For this review, take the finished solid that the model builds, in its own axes (mm). Face numbers are marked on the shaded views. A direction names the side the tool comes from. Round coordinates to 2 decimals unless told otherwise and drop trailing zeros. Write each loop counter-clockwise with the first axis right and the second up, starting at its lowest first coordinate (ties: lowest second). Pieces come first, ordered by that corner, then holes. Notation, with made-up numbers: (79, 67) -> (122, 67) arc R11 ccw to (122, 75) -> close; hole circle Ø3 at (6.5, 85). An arc over 180 degrees is marked (long way). Answer as CSV lines item,"result". Start each with the question number.
Item 1: Take a section at A-A on y = 0. Give the boundary of the cut face in (x, z), then the cut area to 3 significant figures.
Item 2: Wall thickness on probe 1 along Y at (x, z) = (0.5, 2.25); probe 2 along X at (y, z) = (15, 5.25): over which ranges is each line inside the solid? List them lowest first. Write a range as from..to.
Item 3: Machinability: for the marked faces 5 and 6, which of the approach directions +Z, -Z, +X, -X, +Y, -Y give a long, thin tool a straight path to every point of the face, cutting with its end or side? Answer none if there is none.
Item 4: Mouldability with a two-part tool opening along X and no side actions: class the marked faces 1, 2, 3 and 4 as +X half, -X half, draft (parallel to the pull), parting line (faces both ways), or undercut.
Item 5: For pin 1 Ø18.5 at (x, y) = (-3.5, -2) entering from -Z; pin 2 Ø5 at (x, y) = (16, 16) entering from -Z, all flat-tipped, find the tip position at first contact; note any pin that passes through.
Item 6: Take a section at C-C on z = 3. Count the separate pieces of the cut face and the enclosed holes in it, then the cut area to 3 significant figures.
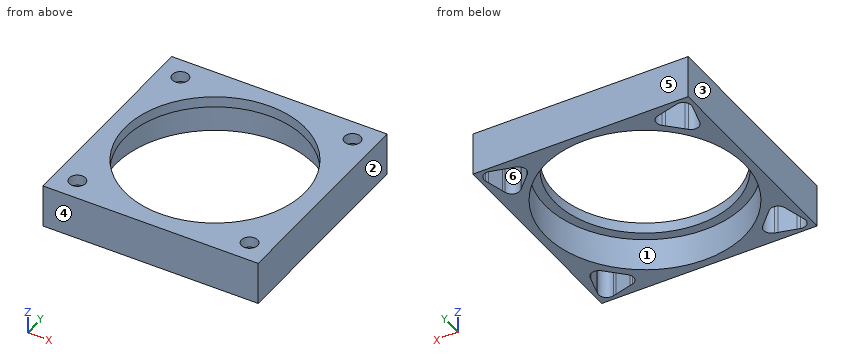
```python
from build123d import *

# Parameters (mm, degrees)
SKETCH_W        = 40
SKETCH_H        = 40
PAD_DEPTH       = 6
POCKET_DEPTH    = 6.001
SKETCH006_R     = 18.5
POCKET001_DEPTH = 6.001
SKETCH007_W     = 40
SKETCH007_H     = 40
SKETCH007_R     = 16.75
SKETCH007_R_2   = 1.5
PAD001_DEPTH    = 2


with BuildPart() as part:
    # Sketch → Pad (new body)
    with BuildSketch(Plane.XY):
        Rectangle(SKETCH_W, SKETCH_H)
    extrude(amount=PAD_DEPTH)

    # Sketch004 (on Face6 of Pad) → Pocket (cut, through all)
    with BuildSketch(Plane.XY.offset(6)):
        with BuildLine():
            Line((12.932774, 15.178139), (15.178139, 12.932774))
            Line((15.178139, 12.932774), (15.586387, 12.524525))
            ThreePointArc((15.586387, 12.524525), (17.035276, 12.136297), (18.095936, 13.196957))
            Line((18.245366, 13.754634), (18.095936, 13.196957))
            Line((18.245366, 13.754634), (19.067226, 16.821861))
            Line((19.067226, 16.821861), (19.216656, 17.379538))
            ThreePointArc((19.216656, 17.379538), (18.828427, 18.828427), (17.379538, 19.216656))
            Line((16.821861, 19.067226), (17.379538, 19.216656))
            Line((16.821861, 19.067226), (13.754634, 18.245366))
            Line((13.754634, 18.245366), (13.196957, 18.095936))
            ThreePointArc((13.196957, 18.095936), (12.136297, 17.035276), (12.524525, 15.586387))
            Line((12.932774, 15.178139), (12.524525, 15.586387))
        make_face()
        with BuildLine():
            Line((13.754634, -18.245366), (16.821861, -19.067226))
            Line((16.821861, -19.067226), (17.379538, -19.216656))
            ThreePointArc((17.379538, -19.216656), (18.828427, -18.828427), (19.216656, -17.379538))
            Line((19.067226, -16.821861), (19.216656, -17.379538))
            Line((19.067226, -16.821861), (18.245366, -13.754634))
            Line((18.245366, -13.754634), (18.095936, -13.196957))
            ThreePointArc((18.095936, -13.196957), (17.035276, -12.136297), (15.586387, -12.524525))
            Line((15.178139, -12.932774), (15.586387, -12.524525))
            Line((15.178139, -12.932774), (12.932774, -15.178139))
            Line((12.932774, -15.178139), (12.524525, -15.586387))
            ThreePointArc((12.524525, -15.586387), (12.136297, -17.035276), (13.196957, -18.095936))
            Line((13.754634, -18.245366), (13.196957, -18.095936))
        make_face()
        with BuildLine():
            Line((-13.754634, 18.245366), (-16.821861, 19.067226))
            Line((-16.821861, 19.067226), (-17.379538, 19.216656))
            ThreePointArc((-17.379538, 19.216656), (-18.828427, 18.828427), (-19.216656, 17.379538))
            Line((-19.067226, 16.821861), (-19.216656, 17.379538))
            Line((-19.067226, 16.821861), (-18.245366, 13.754634))
            Line((-18.245366, 13.754634), (-18.095936, 13.196957))
            ThreePointArc((-18.095936, 13.196957), (-17.035276, 12.136297), (-15.586387, 12.524525))
            Line((-15.178139, 12.932774), (-15.586387, 12.524525))
            Line((-15.178139, 12.932774), (-12.932774, 15.178139))
            Line((-12.932774, 15.178139), (-12.524525, 15.586387))
            ThreePointArc((-12.524525, 15.586387), (-12.136297, 17.035276), (-13.196957, 18.095936))
            Line((-13.754634, 18.245366), (-13.196957, 18.095936))
        make_face()
        with BuildLine():
            Line((-12.932774, -15.178139), (-15.178139, -12.932774))
            Line((-15.178139, -12.932774), (-15.586387, -12.524525))
            ThreePointArc((-15.586387, -12.524525), (-17.035276, -12.136297), (-18.095936, -13.196957))
            Line((-18.245366, -13.754634), (-18.095936, -13.196957))
            Line((-18.245366, -13.754634), (-19.067226, -16.821861))
            Line((-19.067226, -16.821861), (-19.216656, -17.379538))
            ThreePointArc((-19.216656, -17.379538), (-18.828427, -18.828427), (-17.379538, -19.216656))
            Line((-16.821861, -19.067226), (-17.379538, -19.216656))
            Line((-16.821861, -19.067226), (-13.754634, -18.245366))
            Line((-13.754634, -18.245366), (-13.196957, -18.095936))
            ThreePointArc((-13.196957, -18.095936), (-12.136297, -17.035276), (-12.524525, -15.586387))
            Line((-12.932774, -15.178139), (-12.524525, -15.586387))
        make_face()
    extrude(amount=-POCKET_DEPTH, mode=Mode.SUBTRACT)

    # Sketch006 (on Face5 of Pocket) → Pocket001 (cut, through all)
    with BuildSketch(Plane.XY.offset(6)):
        Circle(SKETCH006_R)
    extrude(amount=-POCKET001_DEPTH, mode=Mode.SUBTRACT)

    # Sketch007 (on Face5 of Pocket001) → Pad001 (join)
    with BuildSketch(Plane.XY.offset(6)):
        Rectangle(SKETCH007_W, SKETCH007_H)
        Circle(SKETCH007_R, mode=Mode.SUBTRACT)
        with Locations((-16, 16)):
            Circle(SKETCH007_R_2, mode=Mode.SUBTRACT)
        with Locations((16, 16)):
            Circle(SKETCH007_R_2, mode=Mode.SUBTRACT)
        with Locations((16, -16)):
            Circle(SKETCH007_R_2, mode=Mode.SUBTRACT)
        with Locations((-16, -16)):
            Circle(SKETCH007_R_2, mode=Mode.SUBTRACT)
    extrude(amount=PAD001_DEPTH)


solid = part.part
```
Output values:
1,outline,"(-20, 0) -> (-18.5, 0) -> (-18.5, 6) -> (-16.75, 6) -> (-16.75, 8) -> (-20, 8) -> close; (16.75, 6) -> (18.5, 6) -> (18.5, 0) -> (20, 0) -> (20, 8) -> (16.75, 8) -> close"
1,area,"31.0 mm^2"
2,probe 1,"y = -20..-18.49, 18.49..20"
2,probe 2,"x = -20..-18.58, -13.11..-10.83, 10.83..13.11, 18.58..20"
3,face 5,"+Z, -Z, +X, -X, +Y"
3,face 6,"-Z"
4,face 1,"undercut"
4,face 2,"+X half"
4,face 3,"-X half"
4,face 4,"draft"
5,pin 1,"passes through"
5,pin 2,"stops at z = 6"
6,separate pieces,"1"
6,enclosed holes,"5"
6,area,"386 mm^2"
